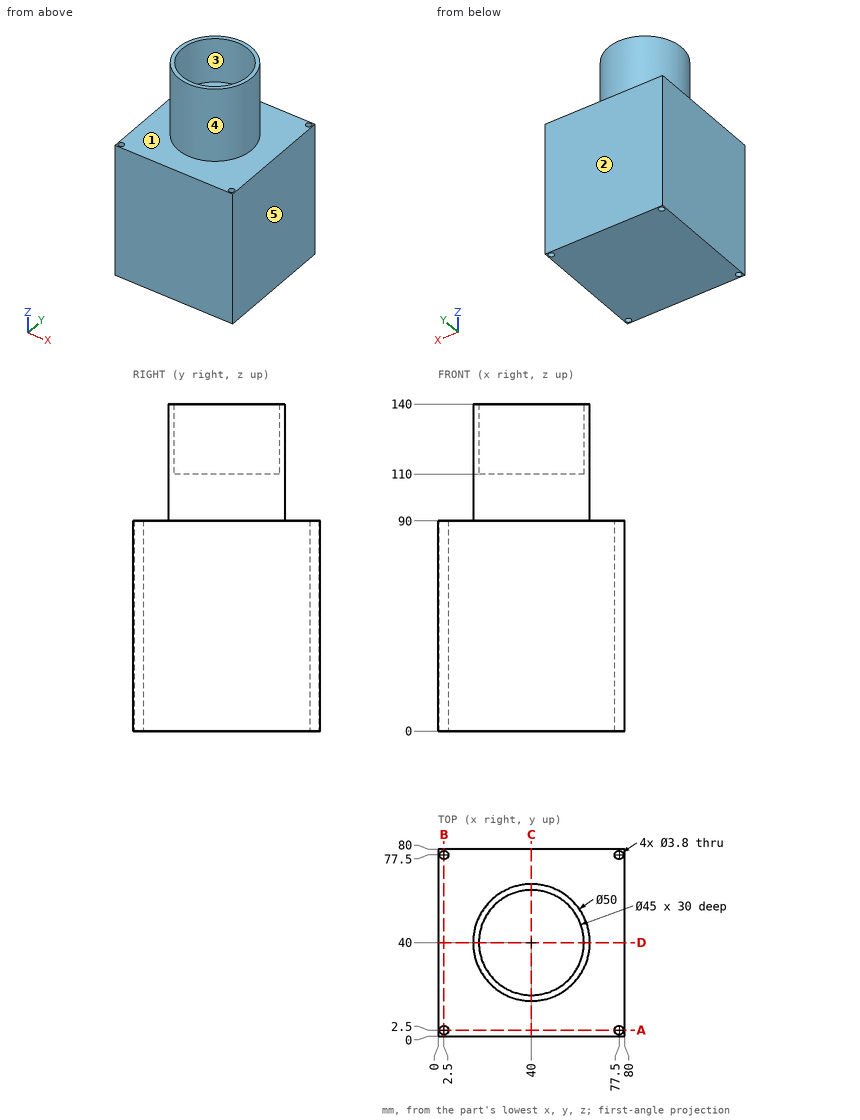
Study the drawing (mm; zero at the part's minimum x, y, z) and answer. A direction names the side the tool comes from. Coordinates: 2 decimals unless noted, no trailing zeros. Loops run counter-clockwise (first coordinate to the right, second up) from the corner with the lowest first, then second, coordinate; pieces in that order, holes last. Notation, with made-up numbers: M 28.5,-23 L 57.5,-23 A25 cw 57.5,-10 Z; hole C 29.25,-14.75 d11. An arc over 180 degrees is marked long. Answer in a Markdown table with one row per item. Add a question column.
1. Find section C-C, the plane x = 40. Write down the section's boundary in (y, z).
2. Consider L1, parallel to Y at x = 77.5, z = 44; L2, parallel to X at y = 77, z = 49; L3, parallel to Z at x = 28, y = 32. Determine where each line is inside the solid, lowest interval first.
3. The mould has two halves that part along Y. Classify the marked faces 1, 2 and 3: pulls with the +Y half, pulls with the -Y half, needs draft (parallel to the pull), parting line crosses it, or undercut.
4. Find section A-A, the plane y = 2.5. Write down the section's boundary in (x, z), then the cut area to 3 significant figures.
5. Flat-ended cylindrical pins translate along their axes: P1, Ø3, axis at x = 2.5, y = 77.5, coming from the +Z side; P2, Ø22.5, axis at x = 32, y = 40.5, coming from the +Z side; P3, Ø1.5, axis at x = 53.5, z = 101.5, coming from the +Y side; P4, Ø4.5, axis at x = 2.5, y = 2.5, coming from the +Z side. Find the tip coordinate at first contact, or state that the pin passes through.
6. A tool of negligible diameter and unlimited length cuts with its end or side. For the marked faces 4 and 5, from which of +Z, -Z, +X, -X, +Y, -Y can it reach the whole face along a straight path? Write none if from no direction.
Reported:
| question | item | result |
|---|---|---|
| 1 | outline | M 0,0 L 80,0 L 80,90 L 65,90 L 65,140 L 62.5,140 L 62.5,110 L 17.5,110 L 17.5,140 L 15,140 L 15,90 L 0,90 Z |
| 2 | L1 | y = 0 to 0.6, 4.4 to 75.6, 79.4 to 80 |
| 2 | L2 | x = 0 to 0.67, 4.33 to 75.67, 79.33 to 80 |
| 2 | L3 | z = 0 to 110 |
| 3 | face 1 | needs draft |
| 3 | face 2 | pulls with the +Y half |
| 3 | face 3 | undercut |
| 4 | outline | M 0,0 L 0.6,0 L 0.6,90 L 0,90 Z; M 4.4,0 L 75.6,0 L 75.6,90 L 4.4,90 Z; M 79.4,0 L 80,0 L 80,90 L 79.4,90 Z |
| 4 | area | 6,520 mm^2 |
| 5 | P1 | passes through |
| 5 | P2 | stops at z = 110 |
| 5 | P3 | stops at y = 61.5 |
| 5 | P4 | stops at z = 90 |
| 6 | face 4 | +Z |
| 6 | face 5 | +Z, -Z, +X, +Y, -Y |
